Verification items for the finished model (mm, model axes). A direction names the side the tool comes from. Coordinates: 2 decimals unless noted, no trailing zeros. Write item = value, one per line.
```python
from build123d import *

# Parameters (mm, degrees)
SKETCH1_R                = 3.1115
BOSS_EXTRUDE1_DEPTH      = 3.81
BOSS_EXTRUDE2_DEPTH      = 5.08
BOSS_EXTRUDE2_DEPTH_BACK = 3.81
BOSS_EXTRUDE3_START      = 0.254
BOSS_EXTRUDE3_DEPTH      = 0.254
BOSS_EXTRUDE4_START      = 2.54
BOSS_EXTRUDE4_DEPTH      = 2.54
BOSS_EXTRUDE5_DEPTH      = 12.7
FILLET1_R                = 7.62
SKETCH11_R               = 2.000000064
CUT_EXTRUDE1_DEPTH       = 6.99999997


with BuildPart() as part:
    # Sketch1 → Boss-Extrude1 (new body)
    with BuildSketch(Plane.XY):
        with BuildLine():
            Line((0, 0), (12.7, 0))
            add(Edge.make_bspline(
                [(0, 12.7), (11.620302725, 11.620302725), (12.7, 0)],
                knots=[0, 0, 0, 1, 1, 1], degree=2))
            Line((0, 12.7), (0, 0))
        make_face()
        with Locations(Location((5.08, 5.08, 0), (0, 0, 180))):
            Circle(SKETCH1_R, mode=Mode.SUBTRACT)
    extrude(amount=BOSS_EXTRUDE1_DEPTH)

    # Sketch2 → Boss-Extrude2 (add, two sides: drawn at the far end of the back side and taken through both)
    with BuildSketch(Plane(origin=(0, 0, 0), x_dir=(-1, 0, 0), z_dir=(0, 0, -1)).offset(-BOSS_EXTRUDE2_DEPTH_BACK)):
        with BuildLine():
            Line((0, 12.7), (1.27, 12.7))
            ThreePointArc((1.27, 12.7), (2.168025612, 12.328025612), (2.54, 11.43))
            Line((2.54, 11.43), (2.54, -1.27))
            ThreePointArc((2.54, -1.27), (2.168025612, -2.168025612), (1.27, -2.54))
            Line((1.27, -2.54), (-11.43, -2.54))
            ThreePointArc((-11.43, -2.54), (-12.328025612, -2.168025612), (-12.7, -1.27))
            Line((-12.7, -1.27), (-12.7, 0))
            Line((-12.7, 0), (0, 0))
            Line((0, 0), (0, 12.7))
        make_face()
    extrude(amount=BOSS_EXTRUDE2_DEPTH + BOSS_EXTRUDE2_DEPTH_BACK)

    # Sketch3 → Boss-Extrude3 (add)
    with BuildSketch(Plane.XY.offset(3.81).offset(BOSS_EXTRUDE3_START)):
        with BuildLine():
            Line((-2.54, 11.43), (-2.54, -1.27))
            ThreePointArc((-2.54, -1.27), (-2.168025612, -2.168025612), (-1.27, -2.54))
            Line((-1.27, -2.54), (11.43, -2.54))
            ThreePointArc((11.43, -2.54), (12.328025612, -2.168025612), (12.7, -1.27))
            Line((12.7, -1.27), (12.7, 0))
            add(Edge.make_bspline(
                [(0, 12.7), (11.620302725, 11.620302725), (12.7, 0)],
                knots=[0, 0, 0, 1, 1, 1], degree=2))
            Line((0, 12.7), (-1.27, 12.7))
            ThreePointArc((-1.27, 12.7), (-2.168025612, 12.328025612), (-2.54, 11.43))
        make_face()
    extrude(amount=-BOSS_EXTRUDE3_DEPTH)

    # Sketch4 → Boss-Extrude4 (add)
    with BuildSketch(Plane.XY.offset(4.064).offset(BOSS_EXTRUDE4_START)):
        with BuildLine():
            Line((-2.54, 11.43), (-2.54, -1.27))
            ThreePointArc((-2.54, -1.27), (-2.168025612, -2.168025612), (-1.27, -2.54))
            Line((-1.27, -2.54), (11.43, -2.54))
            ThreePointArc((11.43, -2.54), (12.328025612, -2.168025612), (12.7, -1.27))
            Line((12.7, -1.27), (12.7, 0))
            add(Edge.make_bspline(
                [(0, 12.7), (11.620302725, 11.620302725), (12.7, 0)],
                knots=[0, 0, 0, 1, 1, 1], degree=2))
            Line((0, 12.7), (-1.27, 12.7))
            ThreePointArc((-1.27, 12.7), (-2.168025612, 12.328025612), (-2.54, 11.43))
        make_face()
    extrude(amount=-BOSS_EXTRUDE4_DEPTH)

    # Sketch10 → Boss-Extrude5 (add)
    with BuildSketch(Plane.ZY.offset(2.54)):
        Polygon((6.604, 11.43), (14.535389884, 5.080302802), (8.339287015, -2.659232815), (6.604, -1.27), align=None)
    extrude(amount=-BOSS_EXTRUDE5_DEPTH)

    # Fillet1
    # the kernel refuses this fillet: 7.62 mm, written as the material it takes off along each edge
    with BuildSketch(Plane(origin=(10.16, 23.335682246, -8.267356033), x_dir=(0, -0.7806486106469015, -0.6249701966454579), z_dir=(0, -0.6249701966454579, 0.7806486106469016))) as fillet1_piece_1_section:
        with BuildLine():
            CenterArc((FILLET1_R, -FILLET1_R), FILLET1_R, 90, 90)
            Line((0, -FILLET1_R), (0, 0))
            Line((0, 0), (FILLET1_R, 0))
        make_face()
    fillet1_piece_1 = extrude(amount=48.26, mode=Mode.PRIVATE)
    fillet1_piece_1 = split(fillet1_piece_1, bisect_by=Plane(origin=(9.16105253, 9.619488642, 6.604), z_dir=(0, 0, 1)), keep=Keep.TOP, mode=Mode.PRIVATE)
    add(fillet1_piece_1, mode=Mode.SUBTRACT)

    # Sketch11 → Cut-Extrude1 (cut)
    with BuildSketch(Plane(origin=(0, -5.107252745, 6.379455822), x_dir=(1, 0, 0), z_dir=(0, -0.6249701966454576, 0.7806486106469017))):
        with Locations(Location((3.81, 8.092998121, 0), (0, 0, 270))):
            Circle(SKETCH11_R)
    extrude(amount=-CUT_EXTRUDE1_DEPTH, mode=Mode.SUBTRACT)


solid = part.part
```
1) Depth check by flat-ended pin: pin 1 Ø5 at (x, y) = (9.5, 7) entering from -Z; pin 2 Ø8 at (y, z) = (6.5, 7.5) entering from +X; pin 3 Ø3 at (x, y) = (10, 10) entering from +Z. Enter the tip coordinate at first touch or a pass-through.
Ans:
pin_1 = 0
pin_2 = 12.3
pin_3 = 6.6
2) Tool access check on faces 1 (the face through (3, 8, 0)), 2 (the face through (10.16, 0, 8)), 3 (the face through (-2.178, -2.158, 0.844)), 4 (the face through (5, 5, 3.81)). Record the directions out of +Z, -Z, +X, -X, +Y, -Y that give a thin tool (end or side, any length) a straight path to the whole face; none if there is none.
Ans:
face_1 = -Z, +X, +Y
face_2 = +Z, +X, +Y, -Y
face_3 = -Z, -X, -Y
face_4 = -Z
3) Material ranges on line 1 (X direction, y = 4, z = -3); line 2 (Z direction, x = 3, y = -1.5); line 3 (Y direction, x = 5.08, z = 1.75), recorded low to high.
Ans:
line_1 = -2.54 to 0
line_2 = -5.08 to 6.6, 6.89 to 9.27
line_3 = -2.54 to 1.97, 8.19 to 11.53
4) Release check for a two-part mould opening along Z. For faces 5 (the face through (12.318, -2.178, 0.844)), 6 (the face through (1.858, 3.706, 9.014)), 7 (the face through (6.98, 6.48, 10.5)) record: pulls with the +Z half, pulls with the -Z half, needs draft (parallel to the pull), parting line crosses it, or undercut.
Ans:
face_5 = needs draft
face_6 = undercut
face_7 = pulls with the +Z half
